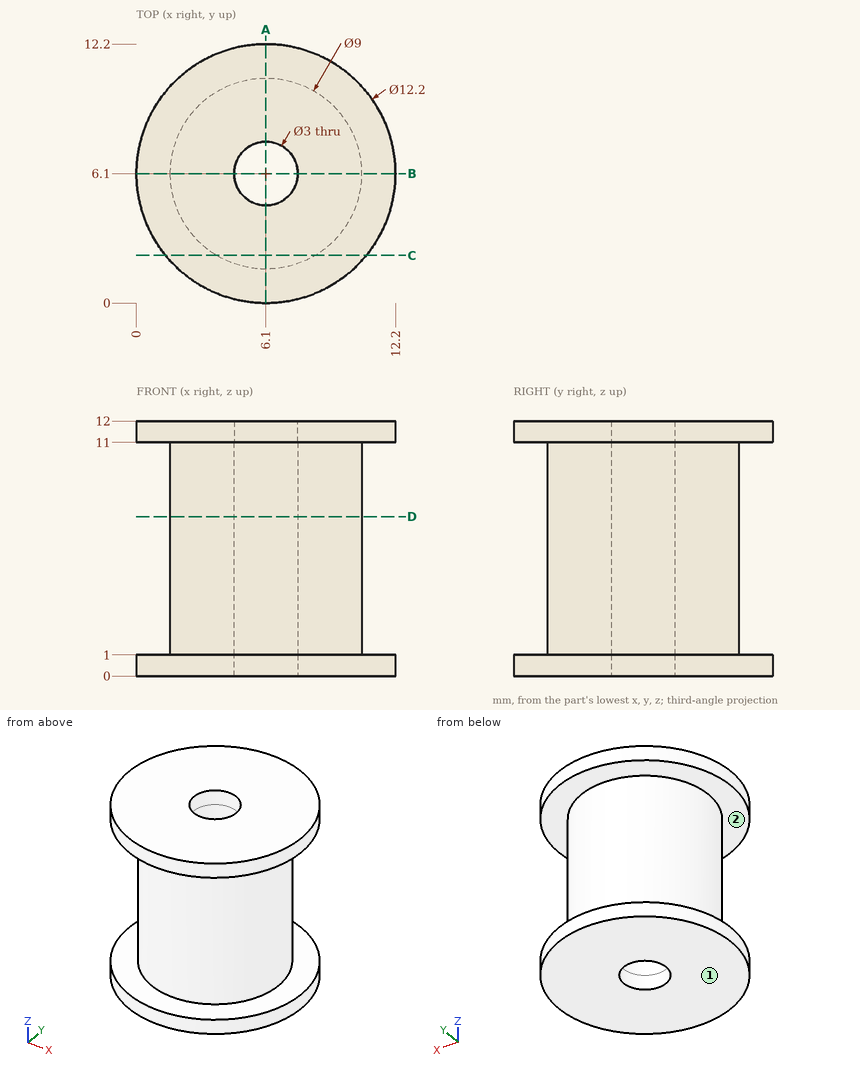
Check sheet for the drawn part. Datum: minimum x, y, z corner. Units: mm. A direction names the side the tool comes from. Round coordinates to 2 decimals unless told otherwise and drop trailing zeros. Loops run counter-clockwise (first coordinate to the right, second up) from the corner with the lowest first, then second, coordinate; pieces in that order, holes last. Notation, with made-up numbers: (21.5, 84.25) - (56.5, 84.25) arc R20 cw to (56.5, 91.25) - close; hole circle Ø11 at (44, 43). An arc over 180 degrees is marked (long way). Answer as a JSON object with one key per item and string values. Group by question number.
Q1. Gauge pin test, flat ends, axial feed: P1, Ø1.8, axis at x = 6.1, y = 6.1, coming from the -Z side; P2, Ø1.5, axis at x = 7.5, z = 10.5, coming from the +Y side; P3, Ø4, axis at x = 6, z = 8, coming from the -Y side; P4, Ø3, axis at x = 1.5, z = 9, coming from the -Y side. Record the tip position at first contact, or that the pin passes through.
Q2. Sectioned sample at A-A, the plane x = 6.1. Enter the section's corners in (y, z), plus the area to 3 significant figures.
Q3. Sectioned sample at D-D, the plane z = 7.5. Enter the section's corners in (x, y).
Q4. Sectioned sample at C-C, the plane y = 2.25. Enter the section's corners in (x, z).
Q5. Scan lines: line 1 along Z through (x, y) = (0.75, 3.5); line 2 along Y through (x, z) = (6.1, 8.75); line 3 along Y through (x, z) = (6.1, 11.6). Record each from-to range of solid material in increasing order. Write a range as [from, to].
Q6. Set-up check for the marked faces 1 and 2: record each of +Z, -Z, +X, -X, +Y, -Y from which the full face is reachable in a straight line by a thin tool's end or side.
Solution:
{
 "1": {"P1": "passes through", "P2": "stops at y = 12.14", "P3": "stops at y = 1.6", "P4": "stops at y = 2.84"},
 "2": {"outline": "(0, 0) - (4.6, 0) - (4.6, 12) - (0, 12) - (0, 11) - (1.6, 11) - (1.6, 1) - (0, 1) - close; (7.6, 0) - (12.2, 0) - (12.2, 1) - (10.6, 1) - (10.6, 11) - (12.2, 11) - (12.2, 12) - (7.6, 12) - close", "area": "78.4 mm²"},
 "3": {"outline": "circle Ø9 at (6.1, 6.1); hole circle Ø3 at (6.1, 6.1)"},
 "4": {"outline": "(1.37, 0) - (10.83, 0) - (10.83, 1) - (8.43, 1) - (8.43, 11) - (10.83, 11) - (10.83, 12) - (1.37, 12) - (1.37, 11) - (3.77, 11) - (3.77, 1) - (1.37, 1) - close"},
 "5": {"line 1": "z = [0, 1], [11, 12]", "line 2": "y = [1.6, 4.6], [7.6, 10.6]", "line 3": "y = [0, 4.6], [7.6, 12.2]"},
 "6": {"face 1": "-Z, +X, -X, +Y, -Y", "face 2": "none"}
}
